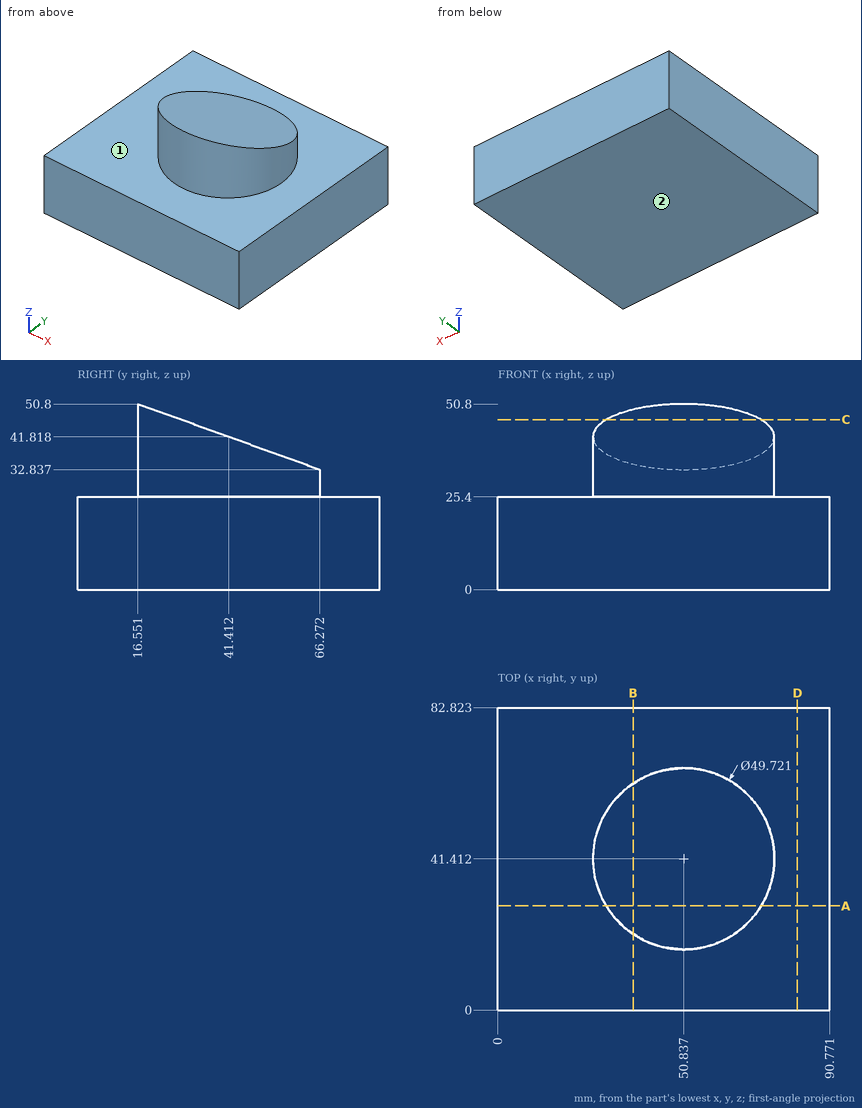
Could you check a few things on this drawing? It's one solid part, dimensions in mm from its lowest x, y, z. A direction names the side the tool comes from. Coordinates: 2 decimals unless noted, no trailing zeros. Order: outer loops, then holes, each group sorted by start corner. A loop starts at its lowest first (then second) coordinate and runs counter-clockwise, first axis right, second up. Notation, with made-up numbers: M 82,13 L 104,13 A22 ccw 104,32 Z; hole C 77.25,69.25 d6. An arc over 180 degrees is marked long. Answer as a JSON object with one key per item and string values. Group by question number.
(1) Suppose I cut it at C-C, the plane z = 46.5. Please give me the cut outline in (x, y), then the cut area to 3 significant figures.
(2) Suppose I cut it at D-D, the plane x = 82. Please give me the cut outline in (y, z), then the cut area to 3 significant figures.
(3) For pin 1 (4 mm diameter, centred on y = 17, z = 29.5, fed in from -X) (1 decimal); pin 2 (2 mm diameter, centred on x = 36, y = 66.5, fed in from +Z); pin 3 (5 mm diameter, centred on y = 27.5, z = 34.5, fed in from -X), each with a flat end and sliding along its axis, tell me the tip position at first contact or that it passes through.
(4) Which directions (+Z, -Z, +X, -X, +Y, -Y) give clear straight access to the entire face, cutting with the end or side of a thin tool? Please do the marked faces 1 and 2.
(5) Suppose I cut it at A-A, the plane y = 28.5. Please give me the cut outline in (x, z), then the cut area to 3 significant figures.
(6) I need wall thicknesses on probe 1 along Z at (x, y) = (49.5, 10); probe 2 along X at (y, z) = (40.5, 27); probe 3 along Z at (x, y) = (68, 31). Which ranges of each line are inside material? Lowest first, please.
(7) Suppose I cut it at B-B, the plane x = 37. Please give me the cut outline in (y, z) (1 decimal), then the cut area to 3 significant figures.
Values found:
{
 "1": {"outline": "M 29.62,28.45 A24.86 ccw 72.05,28.45 Z", "area": "357 mm^2"},
 "2": {"outline": "M 0,0 L 82.82,0 L 82.82,25.4 L 0,25.4 Z", "area": "2,100 mm^2"},
 "3": {"pin 1": "stops at x = 40.1", "pin 2": "stops at z = 25.4", "pin 3": "stops at x = 28.75"},
 "4": {"face 1": "+Z", "face 2": "-Z, +X, -X, +Y, -Y"},
 "5": {"outline": "M 0,0 L 90.77,0 L 90.77,25.4 L 72.08,25.4 L 72.08,46.48 L 29.59,46.48 L 29.59,25.4 L 0,25.4 Z", "area": "3,200 mm^2"},
 "6": {"probe 1": "z = 0 to 25.4", "probe 2": "x = 25.99 to 75.68", "probe 3": "z = 0 to 45.58"},
 "7": {"outline": "M 0,0 L 82.8,0 L 82.8,25.4 L 62.1,25.4 L 62.1,34.4 L 20.8,49.3 L 20.8,25.4 L 0,25.4 Z", "area": "2,780 mm^2"}
}
